Answer from the drawing. Dimensions are ordinates in mm from the lowest x, y and z of the part. Coordinates: 2 decimals unless noted, no trailing zeros. Write each loop counter-clockwise with the first axis right and the second up, starting at its lowest first coordinate (ties: lowest second). Pieces come first, ordered by that corner, then holes.
(1) The part is cut by section A-A, the plane y = 43.5. Determine the outline of the cut face in (x, z).
(2) The part is cut by section C-C, the plane x = 104. Determine the outline of the cut face in (y, z).
(3) The part is cut by section D-D, the plane x = 8. Determine the outline of the cut face in (y, z).
(4) The part is cut by section B-B, the plane z = 32.5. Determine the outline of the cut face in (x, y), and give its area (3 significant figures).
(5) Given pin 1 (8 mm diameter, centred on x = 47, z = 30, fed in from -Y); pin 2 (3 mm diameter, centred on x = 71.5, z = 29.5, fed in from -Y); pin 3 (12 mm diameter, centred on y = 63.5, z = 25, fed in from -X); pin 4 (1.5 mm diameter, centred on x = 108.5, y = 17, fed in from +Z), each flat-ended and moving along its own axis, determine where each tip first touches the part or whether it passes through.
(6) Straight lines are drawn through the part: line 1 along Y through (x, z) = (69, 30.5); line 2 along Z through (x, y) = (96, 86); line 3 along X through (y, z) = (90, 29). For each, find the intervals that lie inside material, in ascending order.
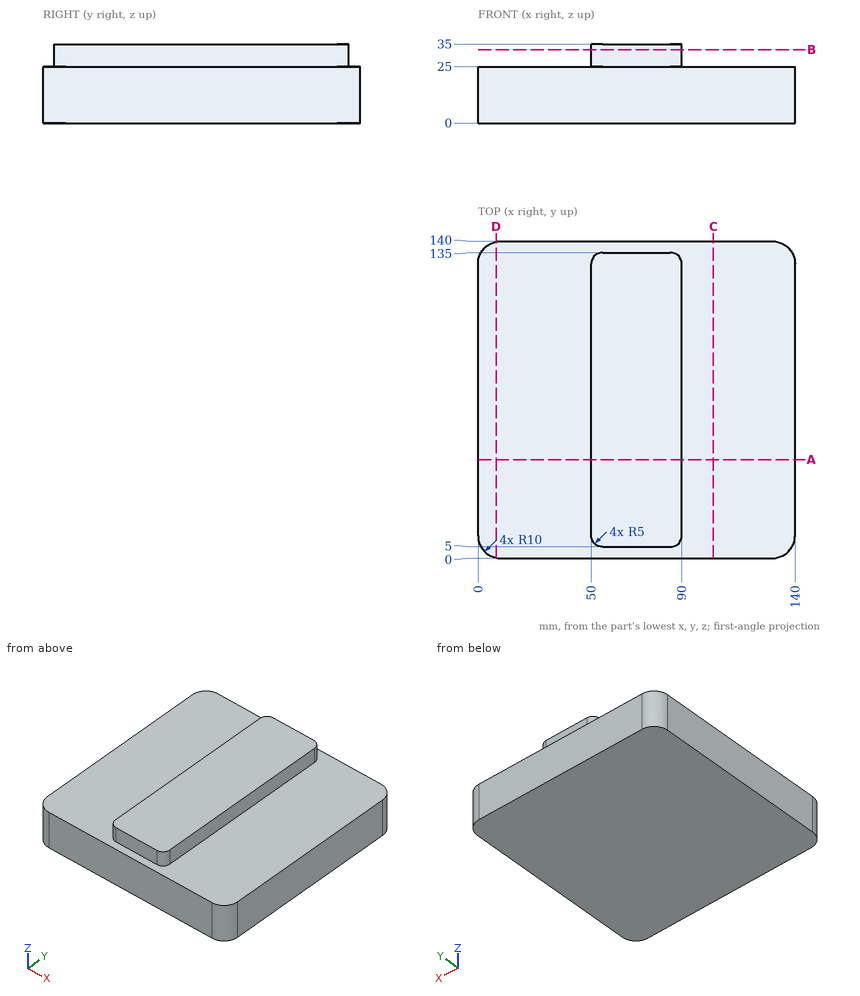
Computed:
1. outline: (0, 0) - (140, 0) - (140, 25) - (90, 25) - (90, 35) - (50, 35) - (50, 25) - (0, 25) - close
2. outline: (0, 0) - (140, 0) - (140, 25) - (0, 25) - close
3. outline: (0.2, 0) - (139.8, 0) - (139.8, 25) - (0.2, 25) - close
4. outline: (50, 10) arc R5 ccw to (55, 5) - (85, 5) arc R5 ccw to (90, 10) - (90, 130) arc R5 ccw to (85, 135) - (55, 135) arc R5 ccw to (50, 130) - close
4. area: 5,180 mm2
5. pin 1: stops at y = 7
5. pin 2: stops at y = 5
5. pin 3: stops at x = 0
5. pin 4: stops at z = 25
6. line 1: y = 5 to 135
6. line 2: z = 0 to 25
6. line 3: x = 50 to 90
